Geometry: see drawing. Coordinates: mm, zero at the bounding-box minimum. Coordinates: 2 decimals unless noted, no trailing zeros. Order: outer loops, then holes, each group sorted by start corner. A loop starts at its lowest first (then second) coordinate and runs counter-clockwise, first axis right, second up. Notation, with made-up numbers: M 55.5,87 L 114.5,87 A33 ccw 114.5,122 Z; hole C 10.5,-4.75 d3. An arc over 180 degrees is marked long. One line per item, written item: value.
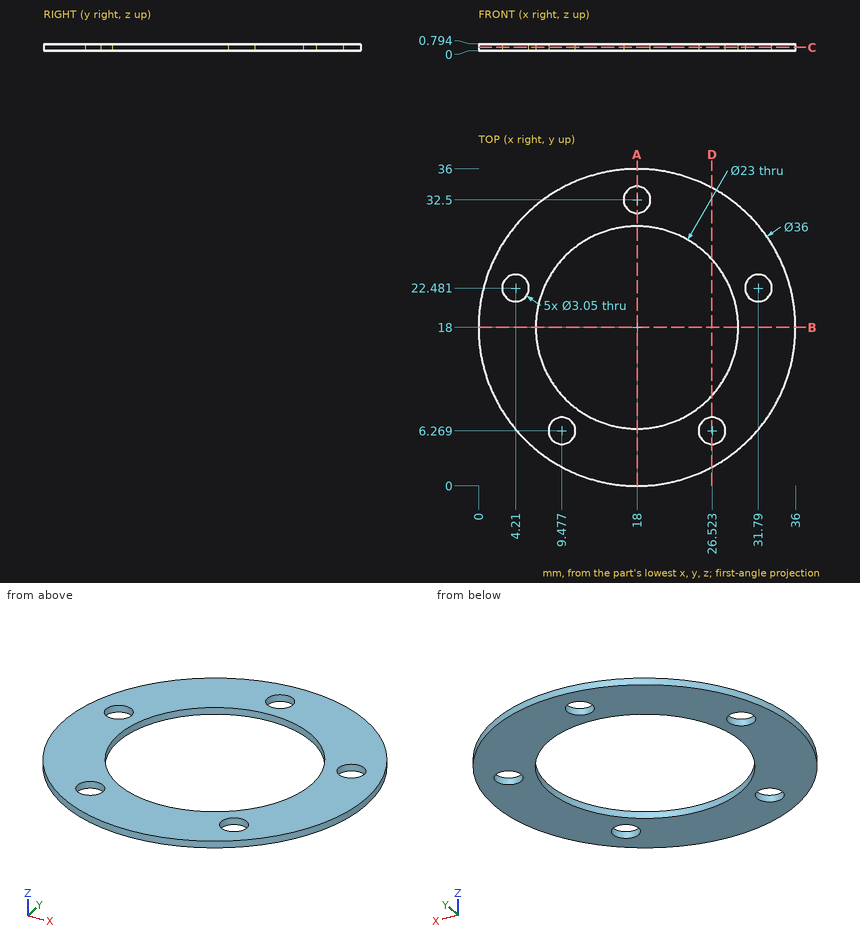
(1) Cut plane D-D on x = 26.5. Output: boundary loops of the cut face in (y, z) (1 decimal).
Data:
outline: M 2.1,0 L 4.7,0 L 4.7,0.8 L 2.1,0.8 Z; M 7.8,0 L 10.3,0 L 10.3,0.8 L 7.8,0.8 Z; M 25.7,0 L 33.9,0 L 33.9,0.8 L 25.7,0.8 Z
(2) Ray query, line 1 (Y direction, x = 18, z = 0.3) (1 decimal); line 2 (Y direction, x = 18.5, z = 0.15); line 3 (Y direction, x = 24, z = 0.35). Return the intervals inside material, ascending. Write a range as from..to.
Data:
line 1: y = 0..6.5, 29.5..31, 34..36
line 2: y = 0.01..6.51, 29.49..31.06, 33.94..35.99
line 3: y = 1.03..8.19, 27.81..34.97
(3) Cut plane C-C on z = 0.4. Give the number of separate pieces and of enclosed holes in the cut face, plus the area to 3 significant figures.
Data:
separate pieces: 1
enclosed holes: 6
area: 566 mm2
(4) Cut plane A-A on x = 18. Output: boundary loops of the cut face in (y, z) (1 decimal).
Data:
outline: M 0,0 L 6.5,0 L 6.5,0.8 L 0,0.8 Z; M 29.5,0 L 31,0 L 31,0.8 L 29.5,0.8 Z; M 34,0 L 36,0 L 36,0.8 L 34,0.8 Z
(5) Cut plane B-B on y = 18. Output: boundary loops of the cut face in (x, z).
Data:
outline: M 0,0 L 6.5,0 L 6.5,0.79 L 0,0.79 Z; M 29.5,0 L 36,0 L 36,0.79 L 29.5,0.79 Z
(6) First-contact query: pin 1 (14 mm diameter, centred on x = 18, y = 18, fed in from -Z); pin 2 (5 mm diameter, centred on x = 9.48, y = 6.27, fed in from +Z). Flat tips, straight axial feed; report the tip coordinate or a pass-through.
Data:
pin 1: passes through
pin 2: stops at z = 0.79
